Check sheet for the drawn part. Datum: minimum x, y, z corner. Units: mm. Round coordinates to 2 decimals unless told otherwise and drop trailing zeros. Write each loop counter-clockwise with the first axis right and the second up, starting at its lowest first coordinate (ties: lowest second). Pieces come first, ordered by that corner, then holes. Notation, with made-up numbers: (37.5, 58.5) - (62.5, 58.5) arc R18 cw to (62.5, 84.5) - close; hole circle Ø11 at (-2, -19). An arc over 180 degrees is marked (long way). Answer as a JSON object with one key per item and string values.
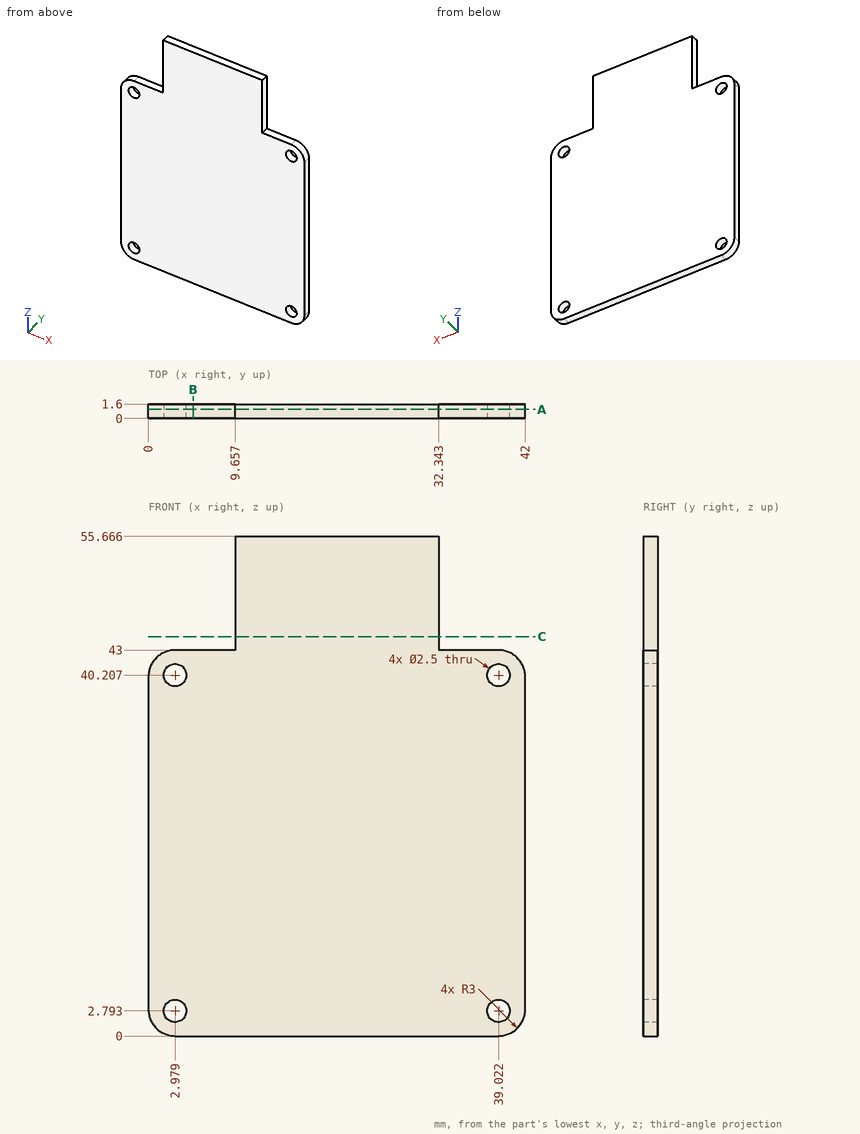
1. Go/stop test with flat-tipped pins: pin 1 (0.5 mm diameter, centred on x = 35.5, y = 1, fed in from +Z); pin 2 (0.5 mm diameter, centred on y = 1, z = 51.5, fed in from +X). Record where each tip stops, or that it passes through.
Completed:
{"pin 1": "stops at z = 43", "pin 2": "stops at x = 32.34"}
2. Cross-section at C-C (z = 44.5). Record the boundary of the cut face in (x, y).
Completed:
{"outline": "(9.66, 0) - (32.34, 0) - (32.34, 1.6) - (9.66, 1.6) - close"}
3. Material ranges on probe 1 along Z at (x, y) = (8.5, 1.5); probe 2 along X at (y, z) = (0.5, 46); probe 3 along Z at (x, y) = (2, 0.3) (1 decimal), recorded low to high. Write a range as from..to.
Completed:
{"probe 1": "z = 0..43", "probe 2": "x = 9.66..32.34", "probe 3": "z = 0.2..2, 3.6..39.4, 41..42.8"}
4. Cross-section at B-B (x = 5). Record the boundary of the cut face in (y, z).
Completed:
{"outline": "(0, 0) - (1.6, 0) - (1.6, 43) - (0, 43) - close"}
5. Cross-section at A-A (y = 1). Record the boundary of the cut face in (x, z).
Completed:
{"outline": "(0, 3) arc R3 ccw to (3, 0) - (39, 0) arc R3 ccw to (42, 3) - (42, 40) arc R3 ccw to (39, 43) - (32.34, 43) - (32.34, 55.67) - (9.66, 55.67) - (9.66, 43) - (3, 43) arc R3 ccw to (0, 40) - close; hole circle Ø2.5 at (2.98, 2.79); hole circle Ø2.5 at (2.98, 40.21); hole circle Ø2.5 at (39.02, 2.79); hole circle Ø2.5 at (39.02, 40.21)"}
